Check sheet for the modelled part. Datum: model origin and axes. Units: mm. Round coordinates to 2 decimals unless told otherwise and drop trailing zeros. Order: outer loops, then holes, each group sorted by start corner. A loop starts at its lowest first (then second) coordinate and runs counter-clockwise, first axis right, second up. Notation, with made-up numbers: (-27.75, 33) -> (-2.75, 33) arc R13 cw to (-2.75, 38) -> close; hole circle Ø5 at (-1, 40.25). An arc over 180 degrees is marked (long way). Answer in a Markdown table with one row per item. Add a question column.
1. Sectioned sample at A-A, the plane z = 0. Record the boundary of the cut face in (x, y).
2. Depth check by flat-ended pin: P1, Ø2, axis at x = 10, y = -177, coming from the -Z side; P2, Ø1, axis at x = 8.5, y = -115.5, coming from the -Z side; P3, Ø2, axis at y = -113, z = 1.5, coming from the +X side; P4, Ø1, axis at y = -161.5, z = -1, coming from the -X side. Enter the tip coordinate at first touch or a pass-through.
3. Material ranges on L1, parallel to Z at x = 8.5, y = -155; L2, parallel to X at y = -185.5, z = 0.1; L3, parallel to X at y = -131.5, z = 0.3, recorded low to high. Write a range as from..to.
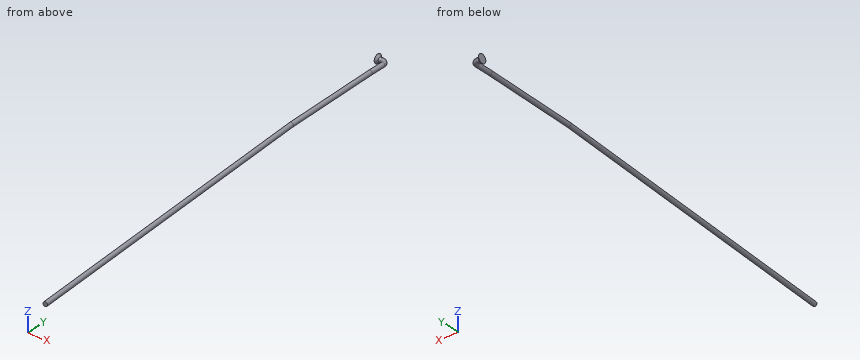
```python
from build123d import *

# Parameters (mm, degrees)
ESQUISSE2_R = 1


with BuildPart() as part:
    # Balayage1: sweep along a path in Esquisse1
    with BuildLine(Plane.XY) as balayage1_path:
        Line((12.227962674, -203.032108123), (1.177962674, -53.984579624))
        Line((1.177962674, -53.984579624), (0, -9))
        Line((0, -9), (0, -2))
        ThreePointArc((0, -2), (-0.585786438, -0.585786438), (-2, 0))
        Line((-2, 0), (-4, 0))
    # Esquisse2 → Balayage1 (sweep)
    with BuildSketch(Plane(origin=(-4, 0, 0), x_dir=(0, 0, -1), z_dir=(1, 0, 0))):
        Circle(ESQUISSE2_R)
    sweep(path=balayage1_path.line, transition=Transition.RIGHT)

    # Esquisse3 → Révolution1 (revolve)
    with BuildSketch(Plane.XY):
        Polygon((-4, 1), (-4, 2), (-3, 1), align=None)
    revolve(axis=Axis((0, 0, 0), (-1, 0, 0)))


solid = part.part
```
Answer key:
| question | item | result |
|---|---|---|
| 1 | outline | (-4, -2) -> (-3, -1) -> (-2, -1) arc R1 cw to (-1, -2) -> (-1, -9.01) -> (0.18, -54.03) -> (11.23, -203.11) -> (13.23, -202.96) -> (2.18, -53.93) -> (1, -8.99) -> (1, -2) arc R3 ccw to (-2, 1) -> (-3, 1) -> (-4, 2) -> close |
| 2 | P1 | stops at z = -1 |
| 2 | P2 | passes through |
| 2 | P3 | stops at x = 6.43 |
| 2 | P4 | stops at x = 8.28 |
| 3 | L1 | z = -0.99..0.99 |
| 3 | L2 | x = 9.93..11.93 |
| 3 | L3 | x = 5.97..7.88 |
